```python
from build123d import *

# Parameters (mm, degrees)
F0_W      = 20
F0_H      = 20
F1_DEPTH  = 20
F2_R      = 2.6
F3_DEPTH  = 1
F4_R      = 2.6
F5_DEPTH  = 1
F6_R      = 2.6
F7_DEPTH  = 1
F8_R      = 2.6
F9_DEPTH  = 1
F10_R     = 2.6
F11_DEPTH = 1
F12_R     = 2.6
F13_DEPTH = 1


with BuildPart() as f1:
    # F0 (on Front) → F1 (new body)
    with BuildSketch(Plane.XZ):
        with Locations((-10, 10)):
            Rectangle(F0_W, F0_H)
    extrude(amount=F1_DEPTH)

    # F2 (on face) → F3 (cut)
    with BuildSketch(Plane.XZ.offset(20)):
        with Locations((-10, 10)):
            Circle(F2_R)
        with Locations((-15, 15)):
            Circle(F2_R)
        with Locations((-5, 15)):
            Circle(F2_R)
        with Locations((-15, 5)):
            Circle(F2_R)
        with Locations((-5, 5)):
            Circle(F2_R)
    extrude(amount=-F3_DEPTH, mode=Mode.SUBTRACT)

    # F4 (on face) → F5 (cut)
    with BuildSketch(Plane.YZ):
        with Locations((-15, 15)):
            Circle(F4_R)
        with Locations((-5, 15)):
            Circle(F4_R)
        with Locations((-15, 5)):
            Circle(F4_R)
        with Locations((-5, 5)):
            Circle(F4_R)
    extrude(amount=-F5_DEPTH, mode=Mode.SUBTRACT)

    # F6 (on face) → F7 (cut)
    with BuildSketch(Plane(origin=(-20, 0, 0), x_dir=(0, -1, 0), z_dir=(-1, 0, 0))):
        with Locations((10, 10)):
            Circle(F6_R)
        with Locations((15, 15)):
            Circle(F6_R)
        with Locations((5, 5)):
            Circle(F6_R)
    extrude(amount=-F7_DEPTH, mode=Mode.SUBTRACT)

    # F8 (on face) → F9 (cut)
    with BuildSketch(Plane(origin=(0, 0, 0), x_dir=(-1, 0, 0), z_dir=(0, 1, 0))):
        with Locations((5, 5)):
            Circle(F8_R)
        with Locations((15, 15)):
            Circle(F8_R)
    extrude(amount=-F9_DEPTH, mode=Mode.SUBTRACT)

    # F10 (on face) → F11 (cut)
    with BuildSketch(Plane(origin=(0, 0, 0), x_dir=(1, 0, 0), z_dir=(0, 0, -1))):
        with Locations((-10, 10)):
            Circle(F10_R)
    extrude(amount=-F11_DEPTH, mode=Mode.SUBTRACT)

    # F12 (on face) → F13 (cut)
    with BuildSketch(Plane.XY.offset(20)):
        with Locations((-3.75, -16.25)):
            Circle(F12_R)
        with Locations((-3.75, -3.75)):
            Circle(F12_R)
        with Locations((-16.25, -16.25)):
            Circle(F12_R)
        with Locations((-16.25, -3.75)):
            Circle(F12_R)
        with Locations((-10, -16.25)):
            Circle(F12_R)
        with Locations((-10, -3.75)):
            Circle(F12_R)
    extrude(amount=-F13_DEPTH, mode=Mode.SUBTRACT)


solid = f1.part
```
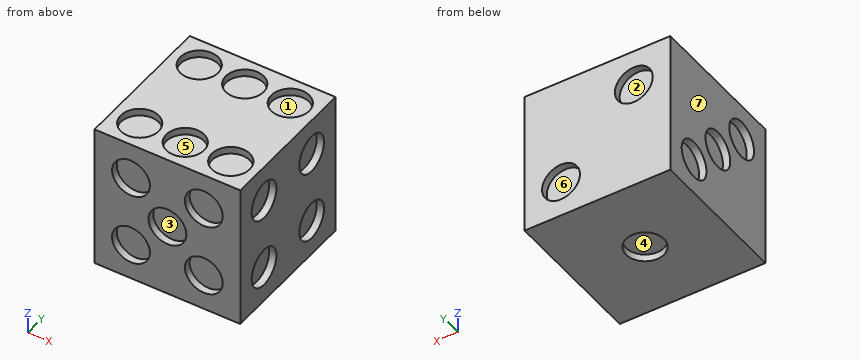
CAD build for the part. Positions are in the model's coordinates, mm. Face numbers are marked on the shaded views. A direction names the side the tool comes from. Coordinates: 2 decimals unless noted, no trailing zeros. Order: outer loops, then holes, each group sorted by start corner. A loop starts at its lowest first (then second) coordinate and runs counter-clockwise, first axis right, second up. Notation, with made-up numbers: M -15,59.25 L -1,59.25 A11 cw -1,79.25 Z; hole C 40,63 d1. An arc over 180 degrees is marked long. Write each question's results on one line, items separated by ' | '. Start each with the question number.
Q1. Cut at D-D (x = -16.25). List the corners of the cut face in (y, z), then the cut area to 3 significant figures.
Q2. Which spindle directions (+Z, -Z, +X, -X, +Y, -Y) get a long thin tool onto all of the face, cutting with end or side? Do the marked faces 1, 2, 3 and 4. Say none if no direction does.
Q3. Drill centre lines: probe 1 along Y at (x, z) = (-10, 19.4); probe 2 along Z at (x, y) = (-19.4, -15); probe 3 along Z at (x, y) = (-19.2, -10). Where is each one in solid material? Low to high. Write a range as from..to.
Q4. Cut at A-A (z = 15). List the corners of the cut face in (x, y), then the cut area to 3 significant figures.
Q5. Cut at B-B (x = -10). List the corners of the cut face in (y, z).
Q6. Cut at C-C (y = -15). List the corners of the cut face in (x, z), then the cut area to 3 significant figures.
Q7. Flat gauge pins, fed straight in: P1, Ø6, axis at y = -4.5, z = 6.5, coming from the -X side; P2, Ø1.6, axis at y = -16, z = 15, coming from the +X side; P3, Ø1.6, axis at x = -6, z = 4, coming from the -Y side; P4, Ø4, axis at x = -16.5, y = -4, coming from the +Z side. Where does each tip first touch, or does it go through?
Q8. Pull direction Z, two halves, no side cores. Call the marked faces 5, 6 and 7: +Z half, -Z half, draft (parallel to the pull), parting line (faces both ways), or undercut.
Found:
1) outline: M -20,0 L 0,0 L 0,12.72 L -1,12.72 L -1,17.28 L 0,17.28 L 0,20 L -1.15,20 L -1.15,19 L -6.35,19 L -6.35,20 L -13.65,20 L -13.65,19 L -18.85,19 L -18.85,20 L -20,20 L -20,17.28 L -19,17.28 L -19,12.72 L -20,12.72 L -20,7.28 L -19,7.28 L -19,2.72 L -20,2.72 Z | area: 376 mm²
2) face 1: +Z | face 2: +Y | face 3: -Y | face 4: -Z
3) probe 1: -20..-18.85, -13.65..-6.35, -1.15..0 | probe 2: 0..12.4, 17.6..20 | probe 3: 0..7.4, 12.6..20
4) outline: M -20,-20 L -17.6,-20 L -17.6,-19 L -12.4,-19 L -12.4,-20 L -7.6,-20 L -7.6,-19 L -2.4,-19 L -2.4,-20 L 0,-20 L 0,-17.6 L -1,-17.6 L -1,-12.4 L 0,-12.4 L 0,-7.6 L -1,-7.6 L -1,-2.4 L 0,-2.4 L 0,0 L -12.4,0 L -12.4,-1 L -17.6,-1 L -17.6,0 L -20,0 L -20,-12.4 L -19,-12.4 L -19,-17.6 L -20,-17.6 Z | area: 369 mm²
5) outline: M -20,0 L -12.6,0 L -12.6,1 L -7.4,1 L -7.4,0 L 0,0 L 0,20 L -1.15,20 L -1.15,19 L -6.35,19 L -6.35,20 L -13.65,20 L -13.65,19 L -18.85,19 L -18.85,20 L -20,20 L -20,12.6 L -19,12.6 L -19,7.4 L -20,7.4 Z
6) outline: M -20,0 L 0,0 L 0,2.4 L -1,2.4 L -1,7.6 L 0,7.6 L 0,12.4 L -1,12.4 L -1,17.6 L 0,17.6 L 0,20 L -1.47,20 L -1.47,19 L -6.03,19 L -6.03,20 L -7.72,20 L -7.72,19 L -12.28,19 L -12.28,20 L -13.97,20 L -13.97,19 L -18.53,19 L -18.53,20 L -20,20 L -20,17.6 L -19,17.6 L -19,12.4 L -20,12.4 Z | area: 371 mm²
7) P1: x = -20 | P2: x = -1 | P3: y = -19 | P4: z = 19
8) face 5: +Z half | face 6: undercut | face 7: draft
